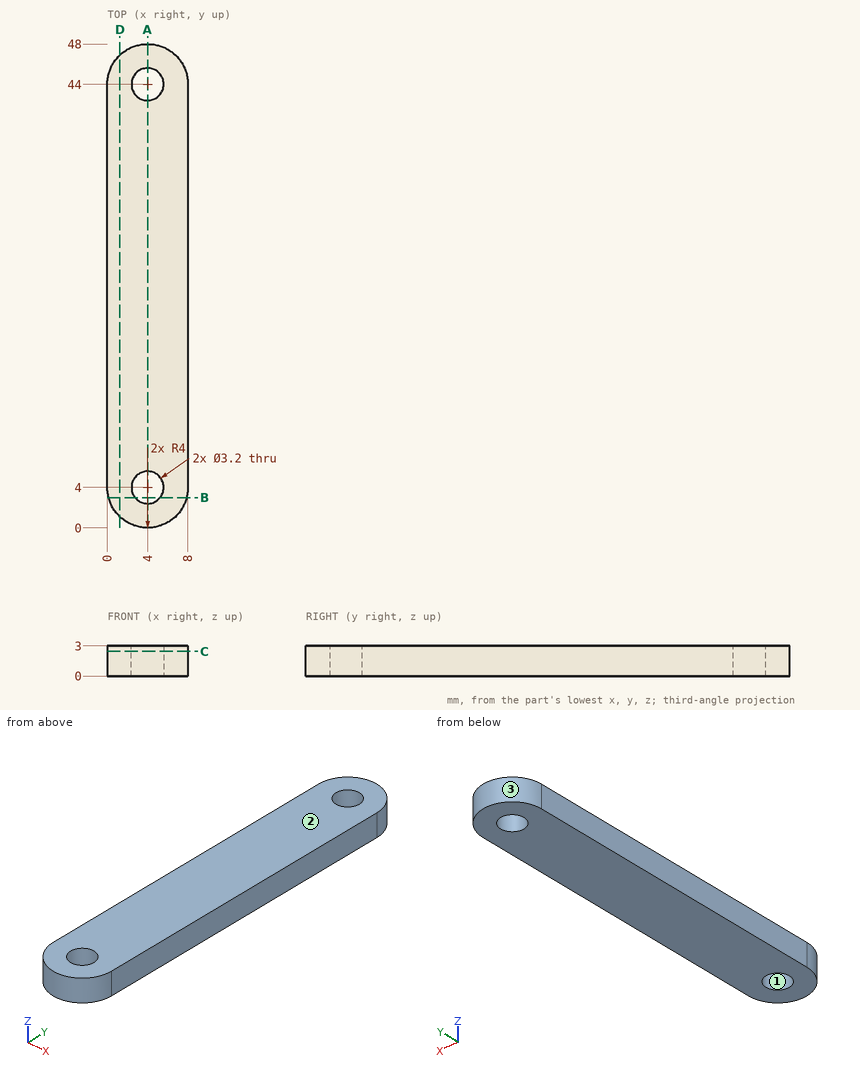
Source: three-view drawing plus pictorial views. Frame: mm from the lowest corner of the part. Round coordinates to 2 decimals unless told otherwise and drop trailing zeros. Loops run counter-clockwise (first coordinate to the right, second up) from the corner with the lowest first, then second, coordinate; pieces in that order, holes last. Notation, with made-up numbers: M 63,31 L 116,31 A20 ccw 116,38 Z; hole C -23,5.25 d9. An arc over 180 degrees is marked long. Answer as CSV lines item,"result". Start each with the question number.
(1) Section D-D, the plane x = 1.25. Output: boundary loops of the cut face in (y, z), plus the area to 3 significant figures.
(2) Draft query along Y for the marked faces 1, 2 and 3. Return one class per face: released by +Y, released by -Y, zero draft, split by the parting line, or undercut.
(3) Section B-B, the plane y = 3. Output: boundary loops of the cut face in (x, z), plus the area to 3 significant figures.
(4) First-contact query: pin 1 (1 mm diameter, centred on y = 31.5, z = 1.5, fed in from -X); pin 2 (2.5 mm diameter, centred on x = 4, y = 44, fed in from -Z). Flat tips, straight axial feed; report the tip coordinate or a pass-through.
(5) Section C-C, the plane z = 2.45. Output: boundary loops of the cut face in (x, y), plus the area to 3 significant figures.
(6) Line query: line 1 (Y direction, x = 4, z = 1.45); line 2 (Y direction, x = 2.75, z = 0.95); line 3 (X direction, y = 43.5, z = 1.9). Output: solid intervals per line, ascending. Write a range as [from, to].
(7) Section A-A, the plane x = 4. Output: boundary loops of the cut face in (y, z).
Values found:
1,outline,"M 1.1,0 L 46.9,0 L 46.9,3 L 1.1,3 Z"
1,area,"137 mm²"
2,face 1,"undercut"
2,face 2,"zero draft"
2,face 3,"released by +Y"
3,outline,"M 0.13,0 L 2.75,0 L 2.75,3 L 0.13,3 Z; M 5.25,0 L 7.87,0 L 7.87,3 L 5.25,3 Z"
3,area,"15.7 mm²"
4,pin 1,"stops at x = 0"
4,pin 2,"passes through"
5,outline,"M 0,4 A4 ccw 8,4 L 8,44 A4 ccw 0,44 Z; hole C 4,4 d3.2; hole C 4,44 d3.2"
5,area,"354 mm²"
6,line 1,"y = [0, 2.4], [5.6, 42.4], [45.6, 48]"
6,line 2,"y = [0.2, 3], [5, 43], [45, 47.8]"
6,line 3,"x = [0, 2.48], [5.52, 8]"
7,outline,"M 0,0 L 2.4,0 L 2.4,3 L 0,3 Z; M 5.6,0 L 42.4,0 L 42.4,3 L 5.6,3 Z; M 45.6,0 L 48,0 L 48,3 L 45.6,3 Z"
